Design review of the part built by this model. Coordinates are the model's own, in mm. A direction names the side the tool comes from. Round coordinates to 2 decimals unless told otherwise and drop trailing zeros. Loops run counter-clockwise (first coordinate to the right, second up) from the corner with the lowest first, then second, coordinate; pieces in that order, holes last. Notation, with made-up numbers: (-17, 65) -> (-3, 65) arc R17 ccw to (-3, 91) -> close; hole circle Ø9 at (-12.5, -40). An arc over 180 degrees is marked (long way). Answer as CSV lines item,"result". Start each with the question number.
```python
from build123d import *

# Parameters (mm, degrees)
EXTRUDE_1_DEPTH     = 80
SKETCH_2_R          = 2.5
CUT_EXTRUDE_1_DEPTH = 10
SKETCH_3_R          = 2.5
SKETCH_3_R_2        = 4
CUT_EXTRUDE_2_DEPTH = 10
CUT_EXTRUDE_3_DEPTH = 30
SKETCH_5_W          = 20
SKETCH_5_H          = 50
CUT_EXTRUDE_4_DEPTH = 10


with BuildPart() as part:
    # Эскиз1 → Бобышка-Вытянуть1 (new body)
    with BuildSketch(Plane(origin=(0, 0, 0), x_dir=(1, 0, 0), z_dir=(0, 1, 0))):
        Polygon((0, 0), (140, 0), (140, 4), (4, 4), (4, 20), (0, 20), (0, 4), align=None)
    extrude(amount=EXTRUDE_1_DEPTH)

    # Эскиз2 → Вырез-Вытянуть1 (cut)
    with BuildSketch(Plane.ZY):
        with Locations((-12, 40)):
            Circle(SKETCH_2_R)
        with Locations((-12, 10)):
            Circle(SKETCH_2_R)
    extrude(amount=-CUT_EXTRUDE_1_DEPTH, mode=Mode.SUBTRACT)

    # Эскиз3 → Вырез-Вытянуть2 (cut)
    with BuildSketch(Plane.XY):
        with Locations((108, 40)):
            Circle(SKETCH_3_R)
        with Locations((108, 10)):
            Circle(SKETCH_3_R)
        with Locations((123, 65)):
            Circle(SKETCH_3_R_2)
    extrude(amount=-CUT_EXTRUDE_2_DEPTH, mode=Mode.SUBTRACT)

    # Эскиз4 → Вырез-Вытянуть3 (cut)
    with BuildSketch(Plane.XY):
        Polygon((0, 50), (60, 50), (100, 80), (0, 80), align=None)
    extrude(amount=-CUT_EXTRUDE_3_DEPTH, mode=Mode.SUBTRACT)

    # Эскиз5 → Вырез-Вытянуть4 (cut)
    with BuildSketch(Plane.XY):
        with Locations((130, 25)):
            Rectangle(SKETCH_5_W, SKETCH_5_H)
    extrude(amount=-CUT_EXTRUDE_4_DEPTH, mode=Mode.SUBTRACT)


solid = part.part
```
Q1. Machinability: for faces 1 (the flat face through (69, 31, 0)), 2 (the cylindrical face through (1.97, 7.56, -12.54)), 3 (the flat face through (23, 50, -3)), 4 (the flat face through (120, 25, -2)), 5 (the flat face through (73, 31, -4)), which of the approach directions +Z, -Z, +X, -X, +Y, -Y give a long, thin tool a straight path to every point of the face, cutting with its end or side? Answer none if there is none.
Q2. Add section B-B, the plane y = 40. Give the boundary of the cut face in (x, z), and give its area (3 significant figures).
Q3. To check wall thickness, follow probe 1 along Y at (x, z) = (108, -2.75); probe 2 along Y at (x, z) = (0.95, -12); probe 3 along Y at (x, z) = (123, -1.75). State the ranges of each line that lie inside material, in increasing order. Write a range as from..to.
Q4. Mouldability with a two-part tool opening along Y and no side actions: class faces 6 (the flat face through (51, 0, -3)), 7 (the flat face through (2, 25, -20)), 8 (the cylindrical face through (122.133, 61.095, -1.972)) as pulls with the +Y half, pulls with the -Y half, needs draft (parallel to the pull), parting line crosses it, or undercut.
Q5. Add section A-A, the plane x = 123. Give the boundary of the cut face in (y, z).
Q6. For pin 1 Ø3 at (x, z) = (57.5, -4) entering from +Y; pin 2 Ø3 at (x, z) = (127.5, -3) entering from -Y; pin 3 Ø3 at (y, z) = (32, -1) entering from +X, all flat-tipped, find the tip position at first contact; note any pin that passes through.
Q7. Add section D-D, the plane y = 62.5. Give the boundary of the cut face in (x, z).
Q8. Add section C-C, the plane x = 108. Give the boundary of the cut face in (y, z), and give its area (3 significant figures).
Worked answers:
1,face 1,"+Z, +X, -X, +Y, -Y"
1,face 2,"+X, -X"
1,face 3,"+Z, -Z, -X, +Y"
1,face 4,"+Z, -Z, +X, -Y"
1,face 5,"-Z, +X, +Y, -Y"
2,outline,"(0, -20) -> (4, -20) -> (4, -14.5) -> (0, -14.5) -> close; (0, -9.5) -> (4, -9.5) -> (4, -4) -> (105.5, -4) -> (105.5, 0) -> (0, 0) -> close; (110.5, -4) -> (120, -4) -> (120, 0) -> (110.5, 0) -> close"
2,area,"504 mm^2"
3,probe 1,"y = 0..7.5, 12.5..37.5, 42.5..80"
3,probe 2,"y = 0..7.5, 12.5..37.5, 42.5..50"
3,probe 3,"y = 50..61, 69..80"
4,face 6,"pulls with the -Y half"
4,face 7,"needs draft"
4,face 8,"undercut"
5,outline,"(50, -4) -> (61, -4) -> (61, 0) -> (50, 0) -> close; (69, -4) -> (80, -4) -> (80, 0) -> (69, 0) -> close"
6,pin 1,"stops at y = 50"
6,pin 2,"stops at y = 50"
6,pin 3,"stops at x = 120"
7,outline,"(76.67, -4) -> (119.88, -4) -> (119.88, 0) -> (76.67, 0) -> close; (126.12, -4) -> (140, -4) -> (140, 0) -> (126.12, 0) -> close"
8,outline,"(0, -4) -> (7.5, -4) -> (7.5, 0) -> (0, 0) -> close; (12.5, -4) -> (37.5, -4) -> (37.5, 0) -> (12.5, 0) -> close; (42.5, -4) -> (80, -4) -> (80, 0) -> (42.5, 0) -> close"
8,area,"280 mm^2"
